Part model, mm, in its own coordinate system. Round coordinates to 2 decimals unless told otherwise and drop trailing zeros. Write each loop counter-clockwise with the first axis right and the second up, starting at its lowest first coordinate (ties: lowest second). Pieces come first, ordered by that corner, then holes.
1) Saw through at B-B on z = 0. Write the cut outline in (x, y).
2) Drill centre lines: L1, parallel to Z at x = 7.5, y = 71; L2, parallel to X at y = 163, z = 0; L3, parallel to X at y = 151, z = -4.5. Where is each one in solid material? Low to high.
3) Flat gauge pins, fed straight in: pin 1 (1 mm diameter, centred on y = 88.5, z = -1, fed in from -X); pin 2 (3 mm diameter, centred on x = -0.5, z = -6, fed in from +Y); pin 3 (1.2 mm diameter, centred on y = 92.5, z = -4, fed in from -X); pin 4 (4.5 mm diameter, centred on x = 1, y = 168.5, fed in from +Z). Where does each tip first touch, or does it go through?
4) Saw through at A-A on x = 0. Write the cut outline in (y, z), and give its area (3 significant figures).
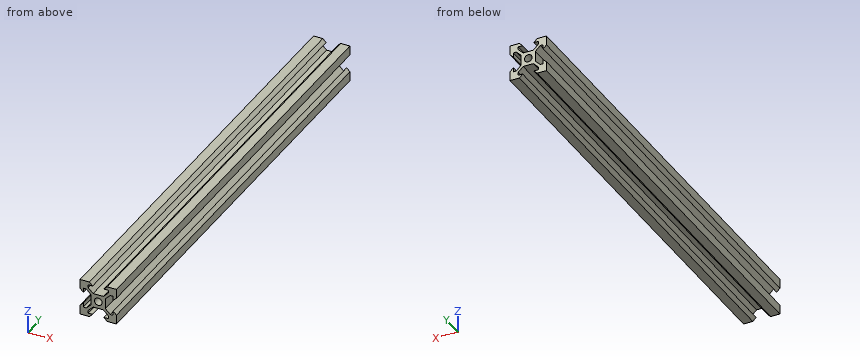
```python
from build123d import *

# Parameters (mm, degrees)
SKETCH1_R           = 2.1
BOSS_EXTRUDE1_DEPTH = 250


with BuildPart() as part:
    # Sketch1 → Boss-Extrude1 (new body)
    with BuildSketch(Plane(origin=(0, 0, 0), x_dir=(1, 0, 0), z_dir=(0, 1, 0))):
        Polygon((-3.900660172, -2.84), (-3.900660172, 0), (-3.900660172, 2.84), (-6.56, 5.499339828), (-8.2, 5.499339828), (-8.2, 3.1), (-10, 4.9), (-10, 10), (-4.9, 10), (-3.1, 8.2), (-5.499339828, 8.2), (-5.499339828, 6.56), (-2.84, 3.900660172), (0, 3.900660172), (2.84, 3.900660172), (5.499339828, 6.56), (5.499339828, 8.2), (3.1, 8.2), (4.9, 10), (10, 10), (10, 4.9), (8.2, 3.1), (8.2, 5.499339828), (6.56, 5.499339828), (3.900660172, 2.84), (3.900660172, 0), (3.900660172, -2.84), (6.56, -5.499339828), (8.2, -5.499339828), (8.2, -3.1), (10, -4.9), (10, -10), (4.9, -10), (3.1, -8.2), (5.499339828, -8.2), (5.499339828, -6.56), (2.84, -3.900660172), (0, -3.900660172), (-2.84, -3.900660172), (-5.499339828, -6.56), (-5.499339828, -8.2), (-3.1, -8.2), (-4.9, -10), (-10, -10), (-10, -4.9), (-8.2, -3.1), (-8.2, -5.499339828), (-6.56, -5.499339828), align=None)
        with Locations(Location((0, 0, 0), (0, 0, 270))):
            Circle(SKETCH1_R, mode=Mode.SUBTRACT)
    extrude(amount=BOSS_EXTRUDE1_DEPTH)


solid = part.part
```
Completed:
1. outline: (-3.9, 0) - (-2.1, 0) - (-2.1, 250) - (-3.9, 250) - close; (2.1, 0) - (3.9, 0) - (3.9, 250) - (2.1, 250) - close
2. L1: z = -10 to -5.5, 5.5 to 10
2. L2: x = -3.9 to -2.1, 2.1 to 3.9
2. L3: x = -9.6 to -8.2, -5.56 to -3.44, 3.44 to 5.56, 8.2 to 9.6
3. pin 1: stops at x = -3.9
3. pin 2: passes through
3. pin 3: stops at x = -9.7
3. pin 4: stops at z = 8.35
4. outline: (0, -3.9) - (250, -3.9) - (250, -2.1) - (0, -2.1) - close; (0, 2.1) - (250, 2.1) - (250, 3.9) - (0, 3.9) - close
4. area: 900 mm2
